Build history of the part. All positions in model axes, mm. A direction names the side the tool comes from. Round coordinates to 2 decimals unless told otherwise and drop trailing zeros. Write each loop counter-clockwise with the first axis right and the second up, starting at its lowest first coordinate (ties: lowest second). Pieces come first, ordered by that corner, then holes. Notation, with made-up numbers: (35.5, 0) - (84.5, 0) arc R15 ccw to (84.5, 28) - close; hole circle Ø2 at (46.25, 35). An arc over 180 degrees is marked (long way). Answer as a JSON object with one key per item and string values. Group by question number.
Item 1: Which spindle directions (+Z, -Z, +X, -X, +Y, -Y) get a long thin tool onto all of the face, cutting with end or side? Do faces 4 (the flat face through (2, -2, -12.7)), 5 (the cylindrical face through (-0.139, 5.078, 5.635)), 6 (the cylindrical face through (-0.44, 1.984, -11.135)). Say none if no direction does.
Item 2: Slice it at A-A, the plane x = 0. Give the number of separate pieces and of enclosed holes in the cut face, then the cut area to 3 significant figures.
Item 3: Probe line 1 (Z direction, x = 0, y = -6.5) (3 decimals); line 2 (Y direction, x = 0, z = -10.9); line 3 (X direction, y = -5.5, z = 6.25). List the from-to ranges inside material, lowest first. Write a range as from..to.
Item 4: Slice it at C-C, the plane z = -10.25. List the corners of the cut face in (x, y), then the cut area to 3 significant figures.
Item 5: Slice it at B-B, the plane z = 1. List the corners of the cut face in (x, y), then the cut area to 3 significant figures.
Item 6: Flat gauge pins, fed straight in: pin 1 (12 mm diameter, centred on x = -6, z = -8, fed in from +Y); pin 2 (5 mm diameter, centred on y = -3.5, z = 2.5, fed in from -X); pin 3 (1.5 mm diameter, centred on x = -4, z = 6, fed in from -Y). Where does each tip first touch, or does it go through?
Item 7: Two-plate mould, pull along Y, no slides. Class faces 1 (the cylindrical face through (0.551, -8.169, 3.235)), 2 (the flat face through (0, -1.906, 3)), 3 (the cylindrical face through (-1.9, 14.48, 5.63)): +Y half, -Y half, draft (parallel to the pull), parting line (faces both ways), or undercut.
from build123d import *

# Parameters (mm, degrees)
F0_R      = 14.604492
F1_DEPTH  = 11.43
F2_R      = 2.54
F3_DEPTH  = 13.6989841001
F5_R      = 7.9375
F6_R      = 14.604492
F8_R      = 1.635125
F9_DEPTH  = 25.4
F8_R_2    = 2.032
F10_DEPTH = 3.175


with BuildPart() as f1:
    # F0 (on Top) → F1 (new body)
    with BuildSketch(Plane.XY):
        Circle(F0_R)
        with BuildLine():
            ThreePointArc((-4.7085324933, -1.905508), (0, 5.079492), (4.7085324933, -1.905508))
            Line((4.7085324933, -1.905508), (-4.7085324933, -1.905508))
        make_face(mode=Mode.SUBTRACT)
    extrude(amount=F1_DEPTH)

    # F2 (on face) → F3 (cut, up to face)
    with BuildSketch(Plane(origin=(0, -1.905508, 0), x_dir=(-1, 0, 0), z_dir=(0, 1, 0))):
        with Locations((0, 5.715)):
            Circle(F2_R)
    extrude(amount=-F3_DEPTH, mode=Mode.SUBTRACT)

    # F5 (on offset) → F7 section 0
    with BuildSketch(Plane.XY.offset(-12.7)):
        Circle(F5_R)
    # F6 (on Top) → F7 section 1
    with BuildSketch(Plane.XY):
        Circle(F6_R)
    loft()

    # F8 (on face) → F9 (cut)
    with BuildSketch(Plane(origin=(0, 0, -12.7), x_dir=(1, 0, 0), z_dir=(0, 0, -1))):
        Circle(F8_R)
    extrude(amount=-F9_DEPTH, mode=Mode.SUBTRACT)

    # F8 (on face) → F10 (cut)
    with BuildSketch(Plane(origin=(0, 0, -12.7), x_dir=(1, 0, 0), z_dir=(0, 0, -1))):
        Circle(F8_R_2)
        Circle(F8_R, mode=Mode.SUBTRACT)
    extrude(amount=-F10_DEPTH, mode=Mode.SUBTRACT)


solid = f1.part
Geometry says:
{
 "1": {"face 4": "-Z, +X, -X, +Y, -Y", "face 5": "+Z", "face 6": "-Z"},
 "2": {"separate pieces": "3", "enclosed holes": "0", "area": "432 mm^2"},
 "3": {"line 1": "z = -12.7..3.175, 8.255..11.43", "line 2": "y = -8.88..-2.03, 2.03..8.88", "line 3": "x = -13.53..-2.48, 2.48..13.53"},
 "4": {"outline": "circle Ø18.45 at (0, 0); hole circle Ø4.06 at (0, 0)", "area": "254 mm^2"},
 "5": {"outline": "circle Ø29.21 at (0, 0); hole (-4.71, -1.91) - (4.71, -1.91) arc R5.08 ccw (long way) to start", "area": "611 mm^2"},
 "6": {"pin 1": "stops at y = 12.8", "pin 2": "stops at x = -14.57", "pin 3": "stops at y = -14.24"},
 "7": {"face 1": "draft", "face 2": "undercut", "face 3": "parting line"}
}
